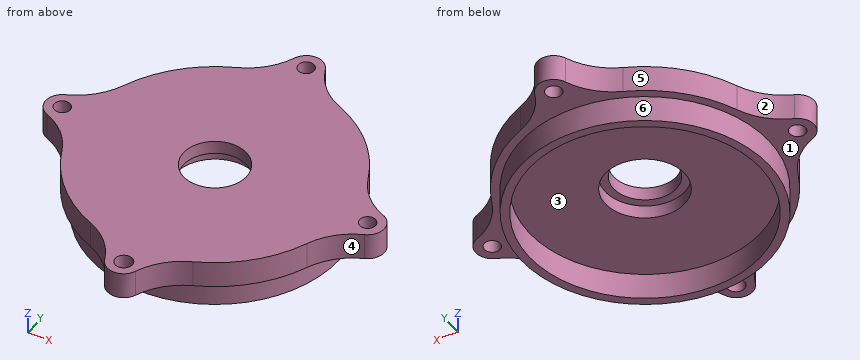
```python
from build123d import *

# Parameters (mm, degrees)
SKETCH_1_R          = 20
EXTRUDE_1_DEPTH     = 4
SKETCH_2_R          = 6
CUT_EXTRUDE_1_DEPTH = 2
SKETCH_3_R          = 4.75
CUT_EXTRUDE_2_DEPTH = 22
SKETCH_4_R          = 18.75
SKETCH_4_R_2        = 17.5
EXTRUDE_2_DEPTH     = 4
SKETCH_5_R          = 1.294929457
SKETCH_5_R_2        = 1.2
EXTRUDE_3_DEPTH     = 4


with BuildPart() as part:
    # 草图1 → 凸台-拉伸1 (new body)
    with BuildSketch(Plane.XY):
        Circle(SKETCH_1_R)
    extrude(amount=EXTRUDE_1_DEPTH)

    # 草图2 → 切除-拉伸1 (cut)
    with BuildSketch(Plane(origin=(0, 0, 0), x_dir=(-1, 0, 0), z_dir=(0, 0, -1))):
        Circle(SKETCH_2_R)
    extrude(amount=-CUT_EXTRUDE_1_DEPTH, mode=Mode.SUBTRACT)

    # 草图3 → 切除-拉伸2 (cut)
    with BuildSketch(Plane.XY.offset(4)):
        Circle(SKETCH_3_R)
    extrude(amount=-CUT_EXTRUDE_2_DEPTH, mode=Mode.SUBTRACT)

    # 草图4 → 凸台-拉伸2 (add)
    with BuildSketch(Plane(origin=(0, 0, 0), x_dir=(-1, 0, 0), z_dir=(0, 0, -1))):
        Circle(SKETCH_4_R)
        Circle(SKETCH_4_R_2, mode=Mode.SUBTRACT)
    extrude(amount=EXTRUDE_2_DEPTH)

    # 草图5 → 凸台-拉伸3 (add)
    with BuildSketch(Plane.XY.offset(4)):
        with BuildLine():
            ThreePointArc((-2.319097331, -23.933695652), (0, -25.5), (2.319097331, -23.933695652))
            ThreePointArc((2.319097331, -23.933695652), (4.474759898, -20.647420615), (7.730324436, -18.445652174))
            ThreePointArc((7.730324436, -18.445652174), (0, -20), (-7.730324436, -18.445652174))
            ThreePointArc((-7.730324436, -18.445652174), (-4.474759898, -20.647420615), (-2.319097331, -23.933695652))
        make_face()
        with Locations((0, -23)):
            Circle(SKETCH_5_R, mode=Mode.SUBTRACT)
        with BuildLine():
            ThreePointArc((-23.933695652, 2.319097331), (-25.5, 0), (-23.933695652, -2.319097331))
            ThreePointArc((-23.933695652, -2.319097331), (-20.647420615, -4.474759898), (-18.445652174, -7.730324436))
            ThreePointArc((-18.445652174, -7.730324436), (-20, 0), (-18.445652174, 7.730324436))
            ThreePointArc((-18.445652174, 7.730324436), (-20.647420615, 4.474759898), (-23.933695652, 2.319097331))
        make_face()
        with Locations((-23, 0)):
            Circle(SKETCH_5_R_2, mode=Mode.SUBTRACT)
        with BuildLine():
            ThreePointArc((23.933695652, -2.319097331), (25.5, 0), (23.933695652, 2.319097331))
            ThreePointArc((23.933695652, 2.319097331), (20.647420615, 4.474759898), (18.445652174, 7.730324436))
            ThreePointArc((18.445652174, 7.730324436), (20, 0), (18.445652174, -7.730324436))
            ThreePointArc((18.445652174, -7.730324436), (20.647420615, -4.474759898), (23.933695652, -2.319097331))
        make_face()
        with Locations((23, 0)):
            Circle(SKETCH_5_R_2, mode=Mode.SUBTRACT)
        with BuildLine():
            ThreePointArc((2.319097331, 23.933695652), (0, 25.5), (-2.319097331, 23.933695652))
            ThreePointArc((-2.319097331, 23.933695652), (-4.474759898, 20.647420615), (-7.730324436, 18.445652174))
            ThreePointArc((-7.730324436, 18.445652174), (0, 20), (7.730324436, 18.445652174))
            ThreePointArc((7.730324436, 18.445652174), (4.474759898, 20.647420615), (2.319097331, 23.933695652))
        make_face()
        with Locations((0, 23)):
            Circle(SKETCH_5_R_2, mode=Mode.SUBTRACT)
    extrude(amount=-EXTRUDE_3_DEPTH)


solid = part.part
```
Work out the finished part from the listing and answer in its coordinate system (mm). Face numbers are marked on the shaded views. A direction names the side the tool comes from. Coordinates: 2 decimals unless noted, no trailing zeros. Order: outer loops, then holes, each group sorted by start corner. A loop starts at its lowest first (then second) coordinate and runs counter-clockwise, first axis right, second up. Notation, with made-up numbers: M -5,33.25 L 47,33.25 A31 ccw 47,72.25 Z; hole C 16.5,53.5 d10. An arc over 180 degrees is marked long. Use CSV: the item, a comma, the result in double quotes.
1) Section C-C on y = -23 is taken. Write down the section's boundary in (x, z).
Worked out:
outline,"M -2.75,0 L -1.29,0 L -1.29,4 L -2.75,4 Z; M 1.29,0 L 2.75,0 L 2.75,4 L 1.29,4 Z"
2) Flat-ended cylindrical pins translate along their axes: pin 1 Ø1.5 at (x, z) = (-17, -2) entering from -Y; pin 2 Ø13 at (x, y) = (0.5, -0.5) entering from -Z; pin 3 Ø1.6 at (x, y) = (0, -23) entering from +Z; pin 4 Ø1 at (x, z) = (-8.5, 0) entering from -Y. Find the tip coordinate at first contact, or state that the pin passes through.
Worked out:
pin 1,"stops at y = -9.35"
pin 2,"stops at z = 0"
pin 3,"passes through"
pin 4,"stops at y = -18.33"
3) Determine the mould class of the marked faces 1, 2, 3 and 4 for opening direction X: released by +X, released by -X, zero draft, split by the parting line, or undercut.
Worked out:
face 1,"zero draft"
face 2,"released by -X"
face 3,"undercut"
face 4,"released by +X"
4) Section A-A on x = 0 is taken. Write down the section's boundary in (y, z), plus the area to 3 significant figures.
Worked out:
outline,"M -25.5,0 L -24.29,0 L -24.29,4 L -25.5,4 Z; M -21.71,0 L -18.75,0 L -18.75,-4 L -17.5,-4 L -17.5,0 L -6,0 L -6,2 L -4.75,2 L -4.75,4 L -21.71,4 Z; M 4.75,2 L 6,2 L 6,0 L 17.5,0 L 17.5,-4 L 18.75,-4 L 18.75,0 L 21.8,0 L 21.8,4 L 4.75,4 Z; M 24.2,0 L 25.5,0 L 25.5,4 L 24.2,4 Z"
area,"151 mm^2"
5) Section B-B on x = 23 is taken. Write down the section's boundary in (y, z).
Worked out:
outline,"M -2.75,0 L -1.2,0 L -1.2,4 L -2.75,4 Z; M 1.2,0 L 2.75,0 L 2.75,4 L 1.2,4 Z"
6) For the marked faces 5 and 6, determine the directions among +Z, -Z, +X, -X, +Y, -Y from which every point of the face is accessible in a straight line to the end or side of a thin tool.
Worked out:
face 5,"+Z, -Z, -X, +Y"
face 6,"-Z"
7) Consider line 1 (Z direction, x = 5, y = 19.5); line 2 (X direction, y = 3, z = -2.25); line 3 (Y direction, x = 0, z = -2.5). Determine where each line is inside the solid, lowest interval first. Write a range as [from, to].
Worked out:
line 1,"z = [0, 4]"
line 2,"x = [-18.51, -17.24], [17.24, 18.51]"
line 3,"y = [-18.75, -17.5], [17.5, 18.75]"
8) Section D-D on z = -3 is taken. Write down the section's boundary in (x, y).
Worked out:
outline,"C 0,0 d37.5; hole C 0,0 d35"
